Geometry: final body of the model. Coordinates: model frame, mm. A direction names the side the tool comes from. Give positions to 0.01 mm unless a question says otherwise; leave off trailing zeros. Write each loop counter-clockwise with the first axis right and the second up, starting at its lowest first coordinate (ties: lowest second). Pieces come first, ordered by that corner, then holes. Notation, with made-up numbers: M -26.75,46 L -4.75,46 A26 ccw -4.75,82 Z; hole C 27.25,-10.75 d6. An arc over 180 degrees is marked long. Use one line per item in the form item = value. Start each with the question number.
Item 1: Section query C-C on x = 32.9. Return loops of the section in (y, z).
Item 2: Pull-direction query (X, two-part tool) for faces 6 (the cylindrical face through (125.67, -100.6, 15.21)), 7 (the flat face through (3, -98, 18)), 8 (the flat face through (124, -1, 35)); classes: released by +X, released by -X, zero draft, split by the parting line, or undercut.
Item 3: Section query A-A on z = 33.5. Return loops of the section in (x, y).
Item 4: Access query for faces 1 (the flat face through (2, -100, 32)), 2 (the flat face through (125, -98, 32)), 3 (the flat face through (62, -49, 0)), 4 (the flat face through (122, -2, 18)), 5 (the flat face through (123, 0, 32)). Directions: +Z, -Z, +X, -X, +Y, -Y. A direction counts if a zero-diameter tool reaches every point of the face in a straight line with its end or side. Return the directions, or none.
Item 5: Material intervals for line 1 along Y through (x, z) = (20, 21); line 2 along X through (y, z) = (-28, 18.5); line 3 along Y through (x, z) = (94, 29), sorted ascending. Write a range as from..to.
Item 6: Contact query for flat-ended pins moving along their axis: P1, Ø1.5, axis at y = -2, z = 33.5, coming from the -X side; P2, Ø1.5, axis at x = 82.5, y = -29, coming from the -Z side; P3, Ø2.5, axis at x = 122.5, z = 33, coming from the -Y side; P4, Ø1.7, axis at y = 1, z = 27.5, coming from the -X side. Output: stop coordinate, or through.
Item 7: Section query B-B on z = 11. Return loops of the section in (x, y), then the cut area to 3 significant figures.
Item 8: Section query D-D on y = -69. Return loops of the section in (x, z), then the cut area to 3 significant figures.
from build123d import *

# Parameters (mm, degrees)
F0_W     = 125
F0_H     = 100
F1_DEPTH = 2
F2_W     = 129.2
F2_H     = 104.2
F2_W_2   = 125
F2_H_2   = 100
F3_DEPTH = 30
F4_R     = 11
F4_W     = 50
F4_H     = 12
F5_DEPTH = 5
F7_DEPTH = 33
F8_R     = 5


with BuildPart() as f1:
    # F0 (on Top) → F1 (new body)
    with BuildSketch(Plane.XY):
        with Locations((62.5, -50)):
            Rectangle(F0_W, F0_H)
    extrude(amount=F1_DEPTH)

    # F2 (on Top) → F3 (join)
    with BuildSketch(Plane.XY):
        with Locations((62.5, -50)):
            Rectangle(F2_W, F2_H)
        with Locations((62.5, -50)):
            Rectangle(F2_W_2, F2_H_2, mode=Mode.SUBTRACT)
    extrude(amount=F3_DEPTH)

    # F4 (on face) → F5 (cut)
    with BuildSketch(Plane(origin=(0, 2.1, 0), x_dir=(-1, 0, 0), z_dir=(0, 1, 0))):
        with Locations((-32.9, 30)):
            Circle(F4_R)
        with Locations((-89.1, 30)):
            Rectangle(F4_W, F4_H)
    extrude(amount=-F5_DEPTH, mode=Mode.SUBTRACT)

    # F6 (on face) → F7 (join)
    with BuildSketch(Plane.XY.offset(2)):
        Polygon((5, 0), (0, 0), (0, -5), align=None)
        Polygon((125, -5), (125, 0), (120, 0), align=None)
        Polygon((120, -100), (125, -100), (125, -95), align=None)
        Polygon((0, -95), (0, -100), (5, -100), align=None)
    extrude(amount=F7_DEPTH)

    # F8
    f8_edges = [f1.edges().sort_by_distance(p)[0] for p in [
        (-2.1, -102.1, 15),
        (127.1, -102.1, 15),
        (127.1, 2.1, 15),
        (-2.1, 2.1, 15),
    ]]
    fillet(f8_edges, radius=F8_R)


solid = f1.part
Answer sheet:
q1.outline = M -102.1,0 L 2.1,0 L 2.1,19 L 0,19 L 0,2 L -100,2 L -100,30 L -102.1,30 Z
q2.face_6 = released by +X
q2.face_7 = undercut
q2.face_8 = zero draft
q3.outline = M 0,-100 L 5,-100 L 0,-95 Z; M 0,-5 L 5,0 L 0,0 Z; M 120,-100 L 125,-100 L 125,-95 Z; M 120,0 L 125,-5 L 125,0 Z
q4.face_1 = +Z, +X, -X, -Y
q4.face_2 = +Z, +X, +Y, -Y
q4.face_3 = -Z, +X, -X, +Y, -Y
q4.face_4 = +Z
q4.face_5 = +Z, +X, -X, +Y
q5.line_1 = -102.1..-100, 0..2.1
q5.line_2 = -2.1..0, 125..127.1
q5.line_3 = -102.1..-100
q6.P1 = 0
q6.P2 = 0
q6.P3 = -100
q6.P4 = -1.06
q7.outline = M -2.1,-97.1 A5 ccw 2.9,-102.1 L 122.1,-102.1 A5 ccw 127.1,-97.1 L 127.1,-2.9 A5 ccw 122.1,2.1 L 2.9,2.1 A5 ccw -2.1,-2.9 Z; hole M 0,-95 L 5,-100 L 120,-100 L 125,-95 L 125,-5 L 120,0 L 5,0 L 0,-5 Z
q7.area = 991 mm2
q8.outline = M -2.1,0 L 127.1,0 L 127.1,30 L 125,30 L 125,2 L 0,2 L 0,30 L -2.1,30 Z
q8.area = 376 mm2
